Source: CAD feature listing. Evaluate the final solid. Frame: model axes, mm. Face numbers are marked on the shaded views. A direction names the side the tool comes from. Round coordinates to 2 decimals unless told otherwise and drop trailing zeros. Order: outer loops, then holes, each group sorted by start corner. A loop starts at its lowest first (then second) coordinate and runs counter-clockwise, first axis right, second up. Notation, with made-up numbers: M 56,5 L 70,5 A8 ccw 70,17 Z; hole C 18,7 d5. An arc over 180 degrees is marked long. Answer as CSV lines item,"result". Start each with the question number.
Item 1: Set-up query: the marked faces 1 and 2. Return all of +Z, -Z, +X, -X, +Y, -Y with unobstructed straight access to the full face (end or side cutting, diameter ignored); none if empty.
Item 2: Pull-direction query (Z, two-part tool) for the marked faces 3, 4 and 5; classes: +Z half, -Z half, draft (parallel to the pull), parting line (faces both ways), or undercut.
Item 3: First-contact query: P1, Ø0.5, axis at y = 12, z = 5, coming from the -X side; P2, Ø0.6, axis at x = -2.5, z = 3, coming from the -Y side; P3, Ø0.8, axis at y = 12, z = 6.5, coming from the +X side. Flat tips, straight axial feed; report the tip coordinate or a pass-through.
Item 4: Line query: line 1 (Z direction, x = -8, y = 7.5); line 2 (Z direction, x = -7.75, y = 9.5); line 3 (X direction, y = 5, z = 7.5). Output: solid intervals per line, ascending. Write a range as [from, to].
Item 5: Section query D-D on x = -5.75. Return the cut outline in (y, z), plus the area to 3 significant figures.
Item 6: Section query A-A on y = 6.5. Return the cut outline in (x, z).
Item 7: Section query C-C on y = 4.5. Return the cut outline in (x, z), plus the area to 3 significant figures.
Item 8: Section query B-B on x = -0.75. Return the cut outline in (y, z), plus the area to 3 significant figures.
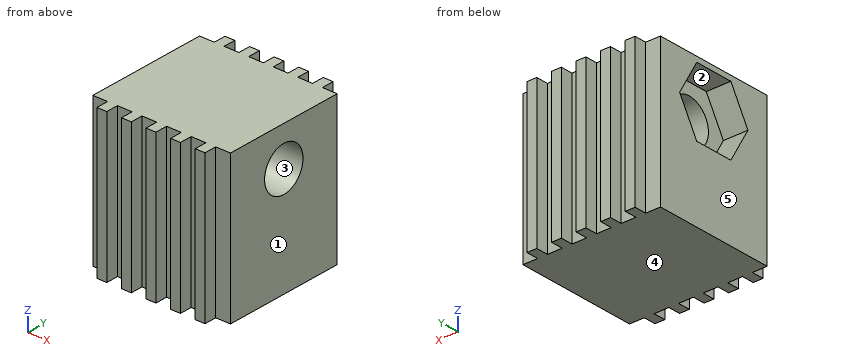
from build123d import *

# Parameters (mm, degrees)
PAD_DEPTH       = 12
SKETCH001_R     = 1.8
POCKET_DEPTH    = 11.201
POCKET001_DEPTH = 3


with BuildPart() as part:
    # Sketch → Pad (new body)
    with BuildSketch(Plane.XY):
        Polygon((-9.211601, 11.50492), (-8.011601, 11.50492), (-8.011601, 12.50492), (-7.211601, 12.50492), (-7.211601, 11.50492), (-6.011601, 11.50492), (-6.011601, 12.50492), (-5.211601, 12.50492), (-5.211601, 11.50492), (-4.011601, 11.50492), (-4.011601, 12.50492), (-3.211601, 12.50492), (-3.211601, 11.50492), (-2.011601, 11.50492), (-2.011601, 12.50492), (-1.211601, 12.50492), (-1.211601, 11.50492), (-0.011601, 11.50492), (-0.011601, 12.50492), (0.788399, 12.50492), (0.788399, 11.50492), (1.988399, 11.50492), (1.988399, 1.50492), (0.788399, 1.50492), (0.788399, 0.50492), (-0.011601, 0.50492), (-0.011601, 1.50492), (-1.211601, 1.50492), (-1.211601, 0.50492), (-2.011601, 0.50492), (-2.011601, 1.50492), (-3.211601, 1.50492), (-3.211601, 0.50492), (-4.011601, 0.50492), (-4.011601, 1.50492), (-5.211601, 1.50492), (-5.211601, 0.50492), (-6.011601, 0.50492), (-6.011601, 1.50492), (-7.211601, 1.50492), (-7.211601, 0.50492), (-8.011601, 0.50492), (-8.011601, 1.50492), (-9.211601, 1.50492), align=None)
    extrude(amount=PAD_DEPTH)

    # Sketch001 → Pocket (cut, through all)
    with BuildSketch(Plane(origin=(-9.211601, 0, 0), x_dir=(0, -1, 0), z_dir=(-1, 0, 0))):
        with Locations((-6.50492, 8.8)):
            Circle(SKETCH001_R)
    extrude(amount=-POCKET_DEPTH, mode=Mode.SUBTRACT)

    # Sketch002 → Pocket001 (cut)
    with BuildSketch(Plane.YZ.offset(-7.211601)):
        Polygon((8.10492, 6.028719), (9.70492, 8.8), (8.10492, 11.571281), (4.90492, 11.571281), (3.30492, 8.8), (4.90492, 6.028719), align=None)
    extrude(amount=-POCKET001_DEPTH, mode=Mode.SUBTRACT)


solid = part.part
Results:
1,face 1,"+Z, -Z, +X, +Y, -Y"
1,face 2,"-X"
2,face 3,"undercut"
2,face 4,"-Z half"
2,face 5,"draft"
3,P1,"x = -8.01"
3,P2,"y = 1.5"
3,P3,"x = 0.79"
4,line 1,"[0, 6.03], [11.57, 12]"
4,line 2,"[0, 8.45], [9.15, 12]"
4,line 3,"[-7.21, 1.99]"
5,outline,"M 0.5,0 L 12.5,0 L 12.5,12 L 0.5,12 Z; hole C 6.5,8.8 d3.6"
5,area,"134 mm^2"
6,outline,"M -9.21,0 L 1.99,0 L 1.99,7 L -7.21,7 L -7.21,6.03 L -9.21,6.03 Z; M -9.21,11.57 L -7.21,11.57 L -7.21,10.6 L 1.99,10.6 L 1.99,12 L -9.21,12 Z"
7,outline,"M -9.21,0 L 1.99,0 L 1.99,12 L -9.21,12 L -9.21,10.87 L -7.21,10.87 L -7.21,6.73 L -9.21,6.73 Z"
7,area,"126 mm^2"
8,outline,"M 1.5,0 L 11.5,0 L 11.5,12 L 1.5,12 Z; hole C 6.5,8.8 d3.6"
8,area,"110 mm^2"
